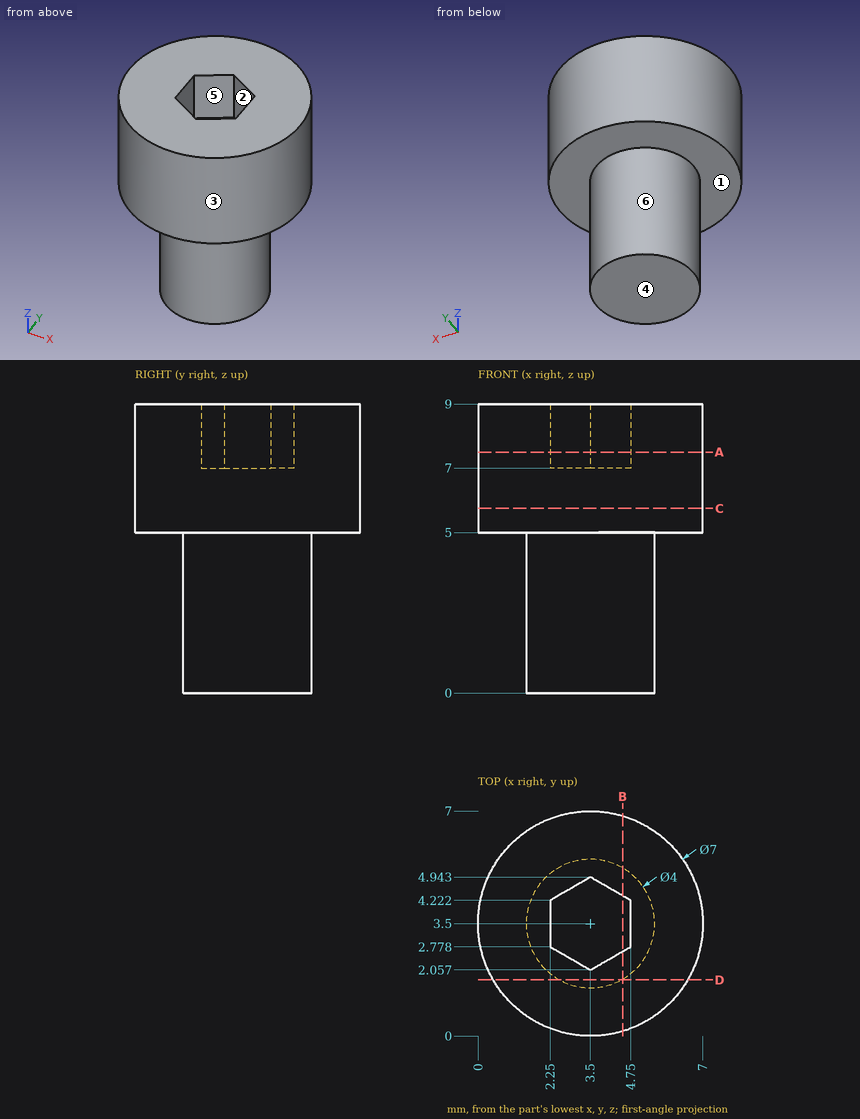
Here's the drawing with two shaded views (mm, measured from the low corner). I have some questions. A direction names the side the tool comes from. Round coordinates to 2 decimals unless told otherwise and drop trailing zeros. Order: outer loops, then holes, each group sorted by start corner. A loop starts at its lowest first (then second) coordinate and runs counter-clockwise, first axis right, second up. Notation, with made-up numbers: (-15.5, -34.5) -> (10.5, -34.5) arc R25 ccw to (10.5, 4.5) -> close; hole circle Ø3 at (40, 32). An arc over 180 degrees is marked (long way). Write each question's results on one line, items separated by ' | '. Start each with the question number.
Item 1: If we section it at A-A, the plane z = 7.5: Write out the boundary of the cut face in (x, y).
Item 2: If we section it at C-C, the plane z = 5.75: Write out the boundary of the cut face in (x, y), then the cut area to 3 significant figures.
Item 3: Will this pin go through, and if not, where does the flat tip stop? pin 1 (2 mm diameter, centred on y = 3, z = 2.5, fed in from -X).
Item 4: Which directions (+Z, -Z, +X, -X, +Y, -Y) give clear straight access to the entire face, cutting with the end or side of a thin tool? Please do the marked faces 4, 5 and 6.
Item 5: Thinking about a two-plate mould opening in X: for the marked faces 1, 2 and 3, which applies, +X half, -X half, draft (parallel to the pull), parting line (faces both ways), or undercut?
Item 6: Please list where these lines run through material, in increasing order: L1, parallel to Z at x = 4.5, y = 1.25; L2, parallel to Y at x = 3, z = 8.5 (1 decimal); L3, parallel to Z at x = 4.5, y = 4.
Item 7: If we section it at B-B, the plane x = 4.5: Write out the boundary of the cut face in (y, z).
Item 8: If we section it at D-D, the plane y = 1.75: Write out the boundary of the cut face in (x, z).
Results:
1) outline: circle Ø7 at (3.5, 3.5); hole (2.25, 2.78) -> (3.5, 2.06) -> (4.75, 2.78) -> (4.75, 4.22) -> (3.5, 4.94) -> (2.25, 4.22) -> close
2) outline: circle Ø7 at (3.5, 3.5) | area: 38.5 mm2
3) pin 1: stops at x = 1.5
4) face 4: -Z, +X, -X, +Y, -Y | face 5: +Z | face 6: -Z
5) face 1: draft | face 2: undercut | face 3: parting line
6) L1: z = 5 to 9 | L2: y = 0 to 2.3, 4.7 to 7 | L3: z = 0 to 7
7) outline: (0.15, 5) -> (1.77, 5) -> (1.77, 0) -> (5.23, 0) -> (5.23, 5) -> (6.85, 5) -> (6.85, 9) -> (4.37, 9) -> (4.37, 7) -> (2.63, 7) -> (2.63, 9) -> (0.15, 9) -> close
8) outline: (0.47, 5) -> (2.53, 5) -> (2.53, 0) -> (4.47, 0) -> (4.47, 5) -> (6.53, 5) -> (6.53, 9) -> (0.47, 9) -> close
